Geometry check sheet. Reference: the model listing, model coordinates, mm. Face numbers are marked on the shaded views. A direction names the side the tool comes from. Give positions to 0.01 mm unless a question says otherwise; leave off trailing zeros. Loops run counter-clockwise (first coordinate to the right, second up) from the corner with the lowest first, then second, coordinate; pieces in that order, holes last. Notation, with made-up numbers: (50.5, 36.25) - (54.5, 36.25) arc R18 ccw to (54.5, 45.25) - close; hole circle Ø10 at (14, 70). An arc over 180 degrees is marked (long way). Write item = value, one per line. Start each with the question number.
Autodesk Inventor part; units mm, degrees
ref_plane "YZ Plane" through (0, 0, 0) normal (1, 0, 0) x (0, 1, 0)
ref_plane "XZ Plane" through (0, 0, 0) normal (0, 1, 0) x (-1, 0, 0)
ref_plane "XY Plane" through (0, 0, 0) normal (0, 0, 1) x (1, 0, 0)
sketch "Sketch1" plane through (0, 0, 0) normal (0, 0, 1) x (1, 0, 0)
  circle A0 centre (0, 0) radius 10.16
  circle A1 centre (0, 0) radius 8.7376
  dimension "d0" = 20.32
  dimension "d6" = 17.4752
extrude "Extrusion1" add sketch "Sketch1" along normal blind 12.7 contours A0 | A1
sketch "Sketch2" plane through (0, 0, 12.7) normal (0, 0, 1) x (1, 0, 0)
  circle A0 centre (0, 0) radius 10.16
  circle A1 centre (0, 0) radius 13.335 construction
  line L0 (0, 13.335) -> (15.875, 13.335)
  line L1 (15.875, 13.335) -> (15.875, -13.335)
  line L2 (15.875, -13.335) -> (0, -13.335)
  arc A2 (0, 13.335) -> (0, -13.335) centre (0, 0) ccw
  point P0 (15.875, 0)
  dimension "d3" = 3.175
  dimension "d14" = 15.875
extrude "Extrusion2" add sketch "Sketch2" along normal blind 6.35 contours A0 | L0 L1 L2 A2
sketch "Sketch4" plane through (0, 0, 19.05) normal (0, 0, 1) x (1, 0, 0)
  arc A0 (0, 13.335) -> (0, -13.335) centre (0, 0) ccw
hole "Hole2" at (0, 0, 19.05) direction (0, 0, -1) diameter 6.5278 end through all
sketch "Sketch5" plane through (0, 0, 19.05) normal (0, 0, 1) x (1, 0, 0)
  line L0 (15.875, 13.335) -> (0, 13.335)
  line L1 (0, -13.335) -> (15.875, -13.335)
  line L2 (15.875, 13.335) -> (9.525, 13.335)
  line L3 (9.525, 13.335) -> (9.525, -13.335)
  line L4 (9.525, -13.335) -> (15.875, -13.335)
  line L5 (15.875, -13.335) -> (15.875, 13.335)
  point P0 (0, 0)
  dimension "d22" = 6.35
extrude "Extrusion3" add sketch "Sketch5" along normal blind 12.7
fillet "Fillet1" radius 3.175 1 edges at (9.525, 0, 19.05)
sketch "Sketch6" plane through (15.875, -13.335, 12.7) normal (1, 0, 0) x (0, 0, -1)
  line L0 (0, 26.67) -> (-19.05, 26.67) construction
  line L1 (-19.05, 0) -> (-19.05, 26.67) construction
  point P0 (12.7, 13.335)
  point P1 (-12.7, 13.335)
  point P2 (-9.525, 26.67)
  point P3 (-19.05, 13.335)
  dimension "d35" = 6.35
hole "Hole3" at (15.875, 0, 25.4) direction (-1, 0, 0) diameter 3.9624 end through all
properties part number "EL2-031" material "ABS Plastic"
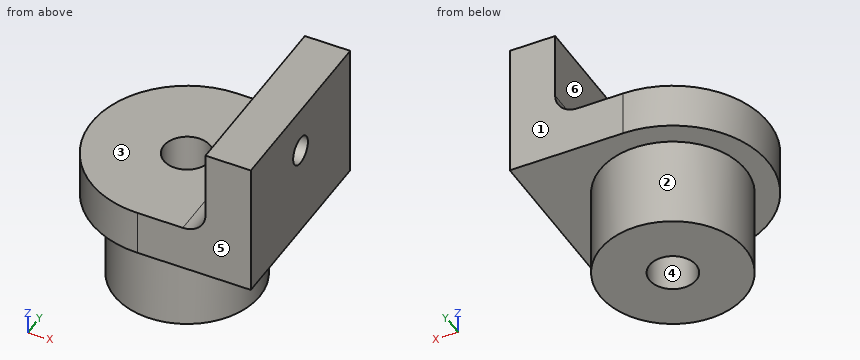
1) Cross-section at D-D on y = -8.75. Enter the section's corners in (x, z) (3 decimals), and give its area (3 significant figures).
2) Material ranges on line 1 along Y through (x, z) = (0, 9.5); line 2 along Z through (x, y) = (12.75, 0); line 3 along X through (y, z) = (-5.25, 25) (3 decimals), recorded low to high.
3) Release check for a two-part mould opening along Y. For the marked faces 4, 5 and 6 record: pulls with the +Y half, pulls with the -Y half, needs draft (parallel to the pull), parting line crosses it, or undercut.
4) Cross-section at C-C on z = 13.5. Enter the section's corners in (x, y) (3 decimals), and give its area (3 significant figures).
5) Cross-section at B-B on y = 0. Enter the section's corners in (x, z) (3 decimals).
6) Gauge pin test, flat ends, axial feed: P1, Ø6, axis at x = 11.5, y = -7.5, coming from the -Z side; P2, Ø6, axis at x = -9, y = -7, coming from the +Z side; P3, Ø1.5, axis at y = -4.5, z = 22, coming from the -X side; P4, Ø5, axis at x = 0, y = 0, coming from the -Z side. Record the tip position at first contact, or that the pin passes through.
7) Cross-section at A-A on z = 25.4. Enter the section's corners in (x, y) (3 decimals).
8) Tool access check on the marked faces 1, 2 and 3. Record the directions out of +Z, -Z, +X, -X, +Y, -Y that give a thin tool (end or side, any length) a straight path to the whole face; none if there is none.
Checked values:
q1.outline = (-10.063, 12.7) - (-5.164, 12.7) - (-5.164, 0) - (5.164, 0) - (5.164, 12.7) - (15.875, 12.7) - (15.875, 31.75) - (9.525, 31.75) - (9.525, 22.225) arc R3.175 cw to (6.35, 19.05) - (-10.063, 19.05) - close
q1.area = 379 mm²
q2.line_1 = -10.16 to -3.26, 3.26 to 10.16
q2.line_2 = 12.7 to 23.42, 27.38 to 31.75
q2.line_3 = 9.525 to 15.875
q3.face_4 = undercut
q3.face_5 = pulls with the -Y half
q3.face_6 = needs draft
q4.outline = (0, -13.335) - (15.875, -13.335) - (15.875, 13.335) - (0, 13.335) arc R13.335 ccw to start; hole circle Ø6.528 at (0, 0)
q4.area = 669 mm²
q5.outline = (-13.335, 12.7) - (-10.16, 12.7) - (-10.16, 0) - (-3.264, 0) - (-3.264, 19.05) - (-13.335, 19.05) - close; (3.264, 0) - (10.16, 0) - (10.16, 12.7) - (15.875, 12.7) - (15.875, 23.419) - (9.525, 23.419) - (9.525, 22.225) arc R3.175 cw to (6.35, 19.05) - (3.264, 19.05) - close; (9.525, 27.381) - (15.875, 27.381) - (15.875, 31.75) - (9.525, 31.75) - close
q6.P1 = 12.7
q6.P2 = 19.05
q6.P3 = 9.37
q6.P4 = through
q7.outline = (9.525, -13.335) - (15.875, -13.335) - (15.875, -1.981) - (9.525, -1.981) - close; (9.525, 1.981) - (15.875, 1.981) - (15.875, 13.335) - (9.525, 13.335) - close
q8.face_1 = +Z, -Z, +X, -X, +Y
q8.face_2 = -Z
q8.face_3 = +Z, -X, +Y, -Y
